Work out the finished part from the listing and answer in its coordinate system (mm). A direction names the side the tool comes from. Coordinates: 2 decimals unless noted, no trailing zeros. Write each loop counter-clockwise with the first axis right and the second up, starting at its lowest first coordinate (ties: lowest second). Pieces come first, ordered by that corner, then holes. Notation, with made-up numbers: M 34.25,55.5 L 84.25,55.5 A31 cw 84.25,93.5 Z; hole C 18.5,31 d9. An arc over 180 degrees is marked long. Answer as CSV lines item,"result". Start each with the question number.
(1) A cutting plane is placed at A-A on x = 156.36. Give the vertices of the cut face in (y, z).
(2) A cutting plane is placed at C-C on x = 425.5. Give the vertices of the cut face in (y, z), then the cut area to 4 significant figures.
(3) The mould has two halves that part along Z. Classify faces 1 (the flat face through (108, 6, 304.8)), 2 (the flat face through (227.79, 9, 85)), 3 (the flat face through (405.39, 6, 318)): released by +Z, released by -Z, zero draft, split by the parting line, or undercut.
(4) A cutting plane is placed at D-D on y = 4.25. Count the separate pieces of the cut face and the enclosed holes in it, then the cut area to 3 significant figures.
(5) Flat-ended cylindrical pins translate along their axes: P1, Ø1.5, axis at y = 8.5, z = 82.5, coming from the -X side; P2, Ø3, axis at x = 153, z = 138, coming from the -Y side; P3, Ø7.5, axis at x = 263, z = 320, coming from the -Y side; P4, Ø2, axis at x = 138.5, y = 13, coming from the -Z side. Find the tip coordinate at first contact, or state that the pin passes through.
(6) For faces 4 (the flat face through (275.59, 6, 318)), 5 (the flat face through (418, 6, 185)), 6 (the flat face through (464, 12.7, 174)), 7 (the flat face through (17.495, 9, 224)), determine the directions among +Z, -Z, +X, -X, +Y, -Y from which every point of the face is accessible in a straight line to the end or side of a thin tool.
(7) Find the intervals of material crossed by L1, parallel to X at y = 16.75, z = 126 (3 decimals); L2, parallel to X at y = 8.5, z = 269.9 (3 decimals); L3, parallel to Z at x = 143.5, y = 7.25, in increasing order. Write a range as [from, to].
Autodesk Inventor part; units mm, degrees
ref_plane "YZ Plane" through (0, 0, 0) normal (1, 0, 0) x (0, 1, 0)
ref_plane "XZ Plane" through (0, 0, 0) normal (0, 1, 0) x (-1, 0, 0)
ref_plane "XY Plane" through (0, 0, 0) normal (0, 0, 1) x (1, 0, 0)
sketch "Sketch1" plane through (0, 0, 0) normal (0, 0, 1) x (1, 0, 0)
  line L0 (0, 0) -> (525.78, 0)
  line L1 (525.78, 0) -> (525.78, 25.4)
  line L2 (525.78, 25.4) -> (0, 25.4)
  line L3 (0, 25.4) -> (0, 0)
  dimension "d0" = 525.78
  dimension "d1" = 25.4
extrude "Extrusion1" add sketch "Sketch1" along normal blind 330.2
sketch "Sketch3" plane through (0, 25.4, 0) normal (0, 1, 0) x (1, 0, 0)
  line L0 (0, -330.2) -> (525.78, -330.2) construction
  line L1 (525.78, -330.2) -> (525.78, -241.3)
  line L2 (525.78, -241.3) -> (0, -241.3) construction
  line L3 (0, -241.3) -> (0, -330.2) construction
  line L4 (86.36, -308.25) -> (86.36, -263.25) construction
  circle A0 centre (86.36, -285.75) radius 2.3812
  circle A1 centre (86.36, -308.25) radius 2.3812
  circle A2 centre (86.36, -263.25) radius 2.3812
  line L5 (146.36, -280.75) -> (146.36, -300.75) construction
  line L6 (156.36, -263.25) -> (156.36, -308.25) construction
  line L7 (146.36, -300.75) -> (166.36, -300.75) construction
  line L8 (166.36, -280.75) -> (146.36, -280.75) construction
  line L9 (86.36, -263.25) -> (226.36, -263.25) construction
  line L10 (226.36, -308.25) -> (86.36, -308.25) construction
  line L11 (86.36, -285.75) -> (226.36, -285.75) construction
  line L12 (166.36, -300.75) -> (166.36, -280.75) construction
  line L13 (226.36, -263.25) -> (226.36, -308.25) construction
  circle A3 centre (226.36, -263.25) radius 2.3813
  circle A4 centre (226.36, -285.75) radius 2.3813
  circle A5 centre (226.36, -308.25) radius 2.3813
  circle A6 centre (156.36, -290.75) radius 10
  line L14 (0, 0) -> (0, -330.2)
  point P0 (525.78, 0)
  point P1 (0, -285.75)
  point P2 (146.36, -290.75)
  point P3 (166.36, -290.75)
  dimension "d16" = 45
  dimension "d17" = 140
  dimension "d18" = 4.7625
  dimension "d19" = 4.7625
  dimension "d20" = 4.7625
  dimension "d21" = 4.7625
  dimension "d22" = 4.7625
  dimension "d23" = 4.7625
  dimension "d24" = 60
  dimension "d25" = 7.5
  dimension "d26" = 20
  dimension "d27" = 20
  dimension "d28" = 86.36
  dimension "d29" = 88.9
extrude "Extrusion3" cut sketch "Sketch3" against normal through all
sketch "Sketch6" plane through (0, 0, 0) normal (0, 0, -1) x (-1, 0, 0)
  line L0 (0, 0) -> (-525.78, 0)
  line L1 (0, 0) -> (-525.78, 0)
  line L2 (-275.59, 0) -> (-250.19, 0)
  line L3 (-250.19, 0) -> (-250.19, 12.7)
  line L4 (-250.19, 12.7) -> (-275.59, 12.7)
  line L5 (-275.59, 12.7) -> (-275.59, 0)
  line L6 (-430.79, 0) -> (-405.39, 0)
  line L7 (-405.39, 0) -> (-405.39, 12.7)
  line L8 (-405.39, 12.7) -> (-430.79, 12.7)
  line L9 (-430.79, 12.7) -> (-430.79, 0)
  line L10 (-120.39, 0) -> (-94.99, 0)
  line L11 (-94.99, 0) -> (-94.99, 12.7)
  line L12 (-94.99, 12.7) -> (-120.39, 12.7)
  line L13 (-120.39, 12.7) -> (-120.39, 0)
  line L14 (-120.39, 6.35) -> (-405.39, 6.35)
  point P0 (-262.89, 0)
  point P1 (-94.99, 6.35)
  point P2 (-262.89, 6.35)
  point P3 (-262.89, 0)
  dimension "d34" = 25.4
  dimension "d35" = 12.7
  dimension "d36" = 25.4
  dimension "d37" = 12.7
  dimension "d40" = 25.4
  dimension "d41" = 12.7
  dimension "d47" = 285
extrude "Extrusion5" cut sketch "Sketch6" against normal blind 185 contours L0 L13 L12 L11 | L0 L5 L14 L3 | L14 L5 L4 L3 | L0 L9 L8 L7
sketch "Sketch8" plane through (0, 0, 330.2) normal (0, 0, 1) x (1, 0, 0)
  line L0 (94.99, 0) -> (120.39, 0)
  line L1 (94.99, 12.7) -> (94.99, 0)
  line L2 (120.39, 12.7) -> (94.99, 12.7)
  line L3 (120.39, 0) -> (120.39, 12.7)
  line L4 (250.19, 0) -> (275.59, 0)
  line L5 (250.19, 12.7) -> (250.19, 0)
  line L6 (275.59, 12.7) -> (250.19, 12.7)
  line L7 (275.59, 0) -> (275.59, 12.7)
  line L8 (405.39, 0) -> (430.79, 0)
  line L9 (405.39, 12.7) -> (405.39, 0)
  line L10 (430.79, 12.7) -> (405.39, 12.7)
  line L11 (430.79, 0) -> (430.79, 12.7)
  point P0 (0, 0)
extrude "Extrusion6" cut sketch "Sketch8" against normal blind 25.4
sketch "Sketch11" plane through (0, 0, 0) normal (0, -1, 0) x (1, 0, 0)
  circle A0 centre (60.195, 317.5) radius 2
  circle A1 centre (185.29, 317.5) radius 2
  circle A2 centre (340.49, 317.5) radius 2
  circle A3 centre (465.585, 317.5) radius 2
  circle A4 centre (465.585, 172.3) radius 2
  circle A5 centre (340.49, 172.3) radius 2
  circle A6 centre (185.29, 172.3) radius 2
  circle A7 centre (60.195, 172.3) radius 2
  line L0 (0, 330.2) -> (94.99, 330.2)
  line L1 (120.39, 330.2) -> (250.19, 330.2)
  line L2 (275.59, 330.2) -> (405.39, 330.2)
  line L3 (430.79, 330.2) -> (525.78, 330.2)
  line L4 (120.39, 304.8) -> (94.99, 304.8)
  line L5 (94.99, 185) -> (120.39, 185)
  point P0 (0, 0)
  point P1 (185.29, 330.2)
  point P2 (340.49, 330.2)
  dimension "d57" = 4
  dimension "d58" = 4
  dimension "d59" = 4
  dimension "d60" = 4
  dimension "d61" = 4
  dimension "d62" = 4
  dimension "d63" = 4
  dimension "d64" = 4
  dimension "d65" = 12.7
  dimension "d66" = 12.7
  dimension "d69" = 60.195
  dimension "d70" = 60.195
extrude "Extrusion8" cut sketch "Sketch11" against normal through all contours A0 | A1 | A3 | A4 | A6 | A7
sketch "Sketch12" plane through (0, 25.4, 0) normal (0, 1, 0) x (1, 0, 0)
  circle A0 centre (60.195, -172.3) radius 2
  circle A1 centre (185.29, -172.3) radius 2
  circle A2 centre (465.585, -172.3) radius 2
  circle A3 centre (465.585, -317.5) radius 2
  circle A4 centre (185.29, -317.5) radius 2
  circle A5 centre (60.195, -317.5) radius 2
  circle A6 centre (60.195, -172.3) radius 2
  circle A7 centre (60.195, -172.3) radius 6.5
  circle A8 centre (60.195, -317.5) radius 2
  circle A9 centre (60.195, -317.5) radius 6.5
  circle A10 centre (185.29, -317.5) radius 2
  circle A11 centre (185.29, -317.5) radius 6.5
  circle A12 centre (185.29, -172.3) radius 2
  circle A13 centre (185.29, -172.3) radius 6.5
  circle A14 centre (465.585, -317.5) radius 6.5
  circle A15 centre (465.585, -172.3) radius 2
  circle A16 centre (465.585, -172.3) radius 6.5
  point P0 (0, 0)
  dimension "d71" = 13
  dimension "d72" = 13
  dimension "d73" = 13
  dimension "d74" = 13
  dimension "d75" = 13
  dimension "d76" = 13
extrude "Extrusion9" cut sketch "Sketch12" against normal blind 12.7 contours A0 | A1 | A2 | A3 | A4 | A5 | A7 | A9 | A11 | A13 | A14 | A16
sketch "Sketch13" plane through (0, 25.4, 0) normal (0, 1, 0) x (1, 0, 0)
  circle A0 centre (349.98, -219.9) radius 4
  circle A1 centre (349.98, -269.9) radius 4
  line L0 (525.78, 0) -> (525.78, -330.2)
  line L1 (525.78, -330.2) -> (0, -330.2)
  point P0 (0, 0)
  dimension "d86" = 8
  dimension "d87" = 8
  dimension "d88" = 175.8
  dimension "d89" = 60.3
  dimension "d90" = 50
extrude "Extrusion10" cut sketch "Sketch13" against normal through all
sketch "Sketch14" plane through (0, 25.4, 0) normal (0, 1, 0) x (1, 0, 0)
  circle A0 centre (349.98, -219.9) radius 4
  circle A1 centre (349.98, -269.9) radius 4
  circle A2 centre (349.98, -219.9) radius 7.5
  circle A3 centre (349.98, -269.9) radius 7.5
  point P0 (0, 0)
  dimension "d93" = 15
  dimension "d94" = 15
extrude "Extrusion11" cut sketch "Sketch14" against normal blind 12.7 contours A0 | A1 | A2 | A3
sketch "Sketch9" plane through (0, 0, 0) normal (0, -1, 0) x (1, 0, 0)
  line L0 (297.99, 146.9) -> (382.99, 146.9)
  line L1 (382.99, 146.9) -> (382.99, 25.4)
  line L2 (382.99, 25.4) -> (297.99, 25.4)
  line L3 (297.99, 25.4) -> (297.99, 146.9)
  line L4 (448.285, 25.4) -> (508.285, 25.4)
  line L5 (508.285, 25.4) -> (508.285, 146.9)
  line L6 (508.285, 146.9) -> (448.285, 146.9)
  line L7 (448.285, 146.9) -> (448.285, 25.4)
  line L8 (142.79, 25.4) -> (227.79, 25.4)
  line L9 (227.79, 25.4) -> (227.79, 146.9)
  line L10 (227.79, 146.9) -> (142.79, 146.9)
  line L11 (142.79, 146.9) -> (142.79, 25.4)
  line L12 (17.495, 25.4) -> (77.495, 25.4)
  line L13 (77.495, 25.4) -> (77.495, 146.9)
  line L14 (77.495, 146.9) -> (17.495, 146.9)
  line L15 (17.495, 146.9) -> (17.495, 25.4)
  line L16 (430.79, 330.2) -> (525.78, 330.2)
  line L17 (275.59, 330.2) -> (405.39, 330.2)
  line L18 (120.39, 0) -> (250.19, 0)
  line L19 (0, 0) -> (94.99, 0)
  line L20 (430.79, 0) -> (525.78, 0)
  circle A0 centre (86.36, 263.25) radius 2.3812
  circle A1 centre (465.585, 172.3) radius 2 construction
  circle A2 centre (465.585, 317.5) radius 2 construction
  line L21 (508.285, 197.7) -> (448.285, 197.7)
  line L22 (448.285, 197.7) -> (448.285, 292.1)
  line L23 (448.285, 292.1) -> (508.285, 292.1)
  line L24 (508.285, 292.1) -> (508.285, 197.7)
  line L25 (382.99, 146.9) -> (297.99, 146.9)
  line L26 (297.99, 146.9) -> (297.99, 292.1)
  line L27 (297.99, 292.1) -> (382.99, 292.1)
  line L28 (382.99, 292.1) -> (382.99, 146.9)
  line L29 (227.79, 210.4) -> (17.495, 210.4)
  line L30 (17.495, 210.4) -> (17.495, 237.85)
  line L31 (17.495, 237.85) -> (227.79, 237.85)
  line L32 (227.79, 237.85) -> (227.79, 210.4)
  line L33 (94.99, 185) -> (120.39, 185)
  line L34 (448.285, 210.4) -> (382.99, 210.4)
  line L35 (382.99, 210.4) -> (382.99, 279.4)
  line L36 (382.99, 279.4) -> (448.285, 279.4)
  line L37 (448.285, 279.4) -> (448.285, 210.4)
  line L38 (430.79, 185) -> (405.39, 185)
  line L39 (405.39, 304.8) -> (430.79, 304.8)
  line L40 (227.79, 210.4) -> (297.99, 210.4)
  line L41 (297.99, 210.4) -> (297.99, 237.85)
  line L42 (297.99, 237.85) -> (227.79, 237.85)
  line L43 (227.79, 237.85) -> (227.79, 210.4)
  point P0 (478.285, 146.9)
  point P1 (478.285, 330.2)
  point P2 (340.49, 146.9)
  point P3 (340.49, 330.2)
  point P4 (185.29, 25.4)
  point P5 (185.29, 0)
  point P6 (47.495, 25.4)
  point P7 (47.495, 0)
  dimension "d48" = 60
  dimension "d49" = 60
  dimension "d50" = 85
  dimension "d51" = 85
  dimension "d53" = 25.4
  dimension "d79" = 25.4
  dimension "d80" = 25.4
  dimension "d81" = 25.4
  dimension "d82" = 25.4
  dimension "d83" = 25.4
  dimension "d84" = 25.4
  dimension "d85" = 25.4
extrude "Extrusion7" cut sketch "Sketch9" against normal blind 19.05 contours L0 L1 L2 L3 | L29 L30 L31 L32 | L22 L23 L24 L21 | L7 L6 L5 L4 | L11 L10 L9 L8 | L15 L14 L13 L12 | A0
sketch "Sketch15" plane through (0, 0, 0) normal (0, 0, -1) x (-1, 0, 0)
  circle A0 centre (-137.795, 12.7) radius 2
  circle A1 centre (-224.3975, 12.7) radius 2
  line L0 (0, 25.4) -> (0, 0)
  line L1 (-525.78, 25.4) -> (0, 25.4)
  line L2 (-262.89, 25.4) -> (-262.89, -36.2644)
  circle A2 centre (-387.985, 12.7) radius 2
  circle A3 centre (-301.3825, 12.7) radius 2
  point P0 (0, 12.7)
  dimension "d97" = 4
  dimension "d98" = 4
  dimension "d99" = 86.6025
  dimension "d100" = 137.795
extrude "Extrusion12" cut sketch "Sketch15" against normal blind 38.1
sketch "Sketch16" plane through (0, 0, 0) normal (0, 0, -1) x (-1, 0, 0)
  circle A0 centre (-50, 12.7) radius 2
  line L0 (0, 25.4) -> (0, 0)
  circle A1 centre (-475.78, 12.7) radius 2
  line L1 (-525.78, 0) -> (-525.78, 25.4)
  point P0 (0, 12.7)
  point P1 (-525.78, 12.7)
  dimension "d103" = 4
  dimension "d104" = 50
  dimension "d105" = 4
  dimension "d106" = 50
extrude "Extrusion13" cut sketch "Sketch16" against normal blind 38.1
properties part number "HB03" material "Polyethylene, High Density"
Here are the results:
1,outline,"M 0,0 L 25.4,0 L 25.4,280.75 L 0,280.75 L 0,237.85 L 19.05,237.85 L 19.05,210.4 L 0,210.4 L 0,146.9 L 19.05,146.9 L 19.05,25.4 L 0,25.4 Z; M 0,300.75 L 25.4,300.75 L 25.4,330.2 L 0,330.2 Z"
2,outline,"M 0,185 L 12.7,185 L 12.7,0 L 25.4,0 L 25.4,330.2 L 12.7,330.2 L 12.7,304.8 L 0,304.8 Z"
2,area,"5,715 mm^2"
3,face 1,"released by +Z"
3,face 2,"undercut"
3,face 3,"zero draft"
4,separate pieces,"1"
4,enclosed holes,"21"
4,area,"110,000 mm^2"
5,P1,"stops at x = 0"
5,P2,"stops at y = 19.05"
5,P3,"stops at y = 12.7"
5,P4,"stops at z = 38.1"
6,face 4,"+Z, -Y"
6,face 5,"-Z, -Y"
6,face 6,"+Y"
6,face 7,"-Y"
7,L1,"x = [0, 17.495], [77.495, 142.79], [227.79, 297.99], [382.99, 448.285], [508.285, 525.78]"
7,L2,"x = [0, 345.98], [353.98, 448.285], [508.285, 525.78]"
7,L3,"z = [0, 25.4], [146.9, 210.4], [237.85, 330.2]"
